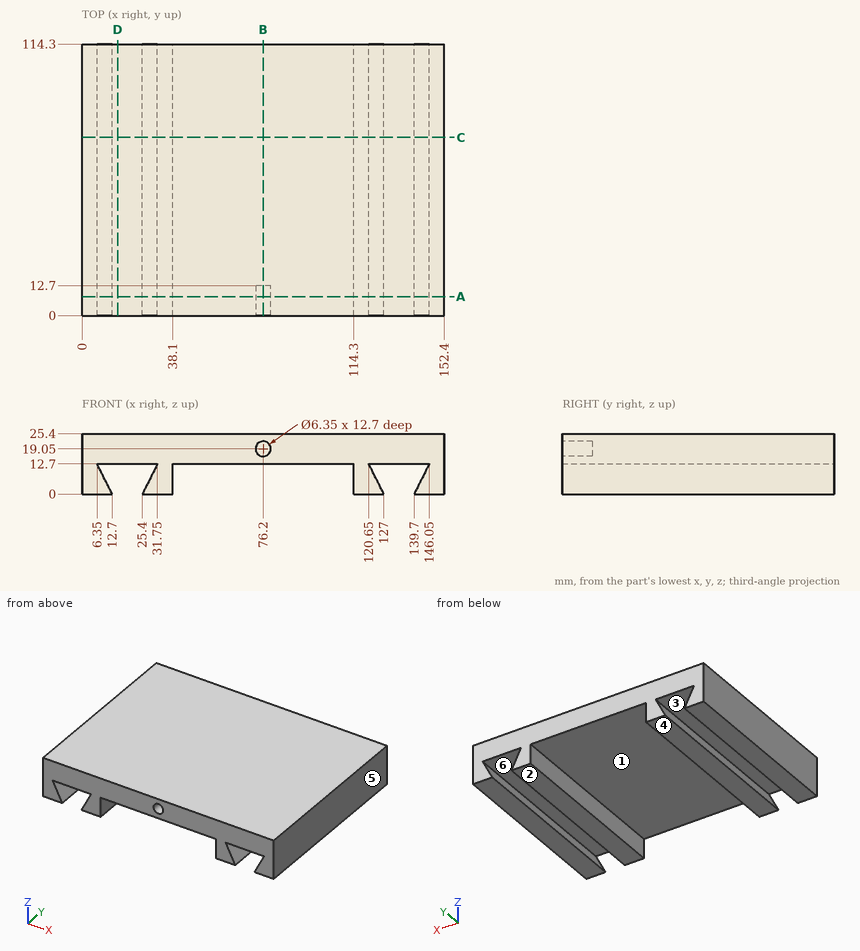
For this review, use the dimensioned drawing (mm, ordinates from the lowest corner) and the shaded views. A direction names the side the tool comes from. Round coordinates to 2 decimals unless told otherwise and drop trailing zeros. Write each loop counter-clockwise with the first axis right and the second up, starting at its lowest first coordinate (ties: lowest second). Pieces come first, ordered by that corner, then holes. Notation, with made-up numbers: M 51.5,33.25 L 57.5,33.25 A9 ccw 57.5,50.25 Z; hole C 58.25,25.25 d6. An arc over 180 degrees is marked long. Answer as CSV lines item,"result". Start each with the question number.
Q1. Wall thickness on line 1 along Z through (x, y) = (76, 3); line 2 along X through (y, z) = (102.5, 1.5); line 3 along X through (y, z) = (86.5, 12): over which ranges is each line inside the solid? List them lowest first.
Q2. Clearance check with a flat-ended pin moving along its axis: P1, Ø1, axis at x = 94.5, y = 50, coming from the -Z side. State where the tip first meets the part, or that it passes through.
Q3. Consider section A-A, the plane y = 8. Give the boundary of the cut face in (x, z) (3 decimals).
Q4. Tool access review of the marked faces 1 and 2: name each direction out of +Z, -Z, +X, -X, +Y, -Y from which nothing blocks a thin tool from reaching the whole face with its end or side.
Q5. Consider section B-B, the plane x = 76.2. Give the boundary of the cut face in (y, z) (3 decimals), then the cut area to 3 significant figures.
Q6. The part is to be moulded in two halves that separate along X. For the marked faces 3, 4, 5 and 6, say which applies: +X half, -X half, draft (parallel to the pull), parting line (faces both ways), or undercut.
Q7. Consider section D-D, the plane x = 15. Give the boundary of the cut face in (y, z), then the cut area to 3 significant figures.
Q8. Consider section C-C, the plane y = 75. Give the boundary of the cut face in (x, z), then the cut area to 3 significant figures.
Result set:
1,line 1,"z = 12.7 to 15.88, 22.22 to 25.4"
1,line 2,"x = 0 to 11.95, 26.15 to 38.1, 114.3 to 126.25, 140.45 to 152.4"
1,line 3,"x = 0 to 6.7, 31.4 to 38.1, 114.3 to 121, 145.7 to 152.4"
2,P1,"stops at z = 12.7"
3,outline,"M 0,0 L 12.7,0 L 6.35,12.7 L 31.75,12.7 L 25.4,0 L 38.1,0 L 38.1,12.7 L 114.3,12.7 L 114.3,0 L 127,0 L 120.65,12.7 L 146.05,12.7 L 139.7,0 L 152.4,0 L 152.4,25.4 L 0,25.4 Z; hole C 76.2,19.05 d6.35"
4,face 1,"-Z, +Y, -Y"
4,face 2,"-Z, +X, -X, +Y, -Y"
5,outline,"M 0,12.7 L 114.3,12.7 L 114.3,25.4 L 0,25.4 L 0,22.225 L 12.7,22.225 L 12.7,15.875 L 0,15.875 Z"
5,area,"1,370 mm²"
6,face 3,"undercut"
6,face 4,"draft"
6,face 5,"+X half"
6,face 6,"undercut"
7,outline,"M 0,12.7 L 114.3,12.7 L 114.3,25.4 L 0,25.4 Z"
7,area,"1,450 mm²"
8,outline,"M 0,0 L 12.7,0 L 6.35,12.7 L 31.75,12.7 L 25.4,0 L 38.1,0 L 38.1,12.7 L 114.3,12.7 L 114.3,0 L 127,0 L 120.65,12.7 L 146.05,12.7 L 139.7,0 L 152.4,0 L 152.4,25.4 L 0,25.4 Z"
8,area,"2,420 mm²"
